```python
from build123d import *

# Parameters (mm, degrees)
VERRUNDUNG1_R = 2


with BuildPart() as part:
    # Skizze1 → Rotation1 (revolve)
    with BuildSketch(Plane.XY, mode=Mode.PRIVATE) as rotation1_sk:
        Polygon((0, 0), (0, 1.267949192), (3, 3), (27, 3), (30, 1.267949192), (30, 0), align=None)
    revolve(rotation1_sk.sketch.rotate(Axis((0, 0, 0), (1, 0, 0)), 180), axis=Axis((0, 0, 0), (1, 0, 0)))

    # Verrundung1
    verrundung1_edges = [part.edges().sort_by_distance(p)[0] for p in [
        (3, 3, 0),
        (27, 3, 0),
    ]]
    fillet(verrundung1_edges, radius=VERRUNDUNG1_R)


solid = part.part
```
Verification items for the finished model (mm, model axes). Coordinates: 2 decimals unless noted, no trailing zeros. Order: outer loops, then holes, each group sorted by start corner. A loop starts at its lowest first (then second) coordinate and runs counter-clockwise, first axis right, second up. Notation, with made-up numbers: (-36.5, -8) -> (14.5, -8) arc R20 cw to (14.5, 7) -> close; hole circle Ø6 at (-26.5, 58). An arc over 180 degrees is marked (long way). Put each result on its own line as item: value. Start each with the question number.
1) Cross-section at A-A (x = 24.5). Enter the section's corners in (y, z).
2) Material ranges on L1, parallel to Z at x = 7, y = -0.2; L2, parallel to Y at x = 10, z = -1.25; L3, parallel to Y at x = 11.5, z = -0.85, recorded low to high.
3) Go/stop test with flat-tipped pins: pin 1 (2 mm diameter, centred on x = 3.5, z = 2.5, fed in from +Y); pin 2 (2 mm diameter, centred on x = 21, z = -1, fed in from +Y); pin 3 (1.5 mm diameter, centred on y = -0.5, z = 2, fed in from -X); pin 4 (1 mm diameter, centred on x = 17, z = 1.5, fed in from -Y). Record where each tip stops, or that it passes through.
4) Cross-section at B-B (x = 28). Enter the section's corners in (y, z).
Geometry check:
1. outline: circle Ø6 at (0, 0)
2. L1: z = -2.99 to 2.99
2. L2: y = -2.73 to 2.73
2. L3: y = -2.88 to 2.88
3. pin 1: stops at y = 2.6
3. pin 2: stops at y = 3
3. pin 3: stops at x = 0.08
3. pin 4: stops at y = -2.83
4. outline: circle Ø4.85 at (0, 0)
